Could you check a few things on this model? Use its own coordinates, in mm. A direction names the side the tool comes from. Coordinates: 2 decimals unless noted, no trailing zeros. Write each loop counter-clockwise with the first axis right and the second up, starting at its lowest first coordinate (ties: lowest second). Pieces come first, ordered by that corner, then holes. Notation, with made-up numbers: M 63,70 L 72,70 A26 ccw 72,86 Z; hole C -3,-19 d7. An arc over 180 degrees is marked long. Write item = value, one per line.
```python
from build123d import *

# Parameters (mm, degrees)
F0_W      = 25
F0_H      = 24
F1_DEPTH  = 1
F2_W      = 8
F2_H      = 8
F3_DEPTH  = 4
F5_DEPTH  = 1
F6_R      = 3.0075631212
F6_R_2    = 1.5783263093
F7_DEPTH  = 1
F8_W      = 21
F8_H      = 6
F9_DEPTH  = 3
F10_W     = 17
F10_H     = 0.5
F11_DEPTH = 3
F2_R      = 0.75
F12_DEPTH = 1


with BuildPart() as f1:
    # F0 (on Top) → F1 (new body)
    with BuildSketch(Plane.XY):
        Rectangle(F0_W, F0_H)
    extrude(amount=F1_DEPTH)

    # F2 (on face) → F3 (join)
    with BuildSketch(Plane.XY.offset(1)):
        with Locations((0, 2.5)):
            Rectangle(F2_W, F2_H)
    extrude(amount=F3_DEPTH)

    # F4 (on face) → F5 (cut)
    with BuildSketch(Plane.XY.offset(5)):
        with BuildLine():
            ThreePointArc((0, 6.5), (2.8284271247, 5.3284271247), (4, 2.5))
            Line((4, 2.5), (4, 6.5))
            Line((4, 6.5), (0, 6.5))
        make_face()
        with BuildLine():
            ThreePointArc((-4, 2.5), (-2.8284271247, 5.3284271247), (0, 6.5))
            Line((0, 6.5), (-4, 6.5))
            Line((-4, 6.5), (-4, 2.5))
        make_face()
        with BuildLine():
            Line((-4, -1.5), (0, -1.5))
            ThreePointArc((0, -1.5), (-2.8284271247, -0.3284271247), (-4, 2.5))
            Line((-4, 2.5), (-4, -1.5))
        make_face()
        with BuildLine():
            Line((4, -1.5), (4, 2.5))
            ThreePointArc((4, 2.5), (2.8284271247, -0.3284271247), (0, -1.5))
            Line((0, -1.5), (4, -1.5))
        make_face()
    extrude(amount=-F5_DEPTH, mode=Mode.SUBTRACT)

    # F6 (on face) → F7 (join)
    with BuildSketch(Plane.XY.offset(5)):
        with Locations((0, 2.5)):
            Circle(F6_R)
        with Locations((0, 2.5)):
            Circle(F6_R_2, mode=Mode.SUBTRACT)
    extrude(amount=F7_DEPTH)

    # F8 (on face) → F9 (join)
    with BuildSketch(Plane(origin=(0, 0, 0), x_dir=(1, 0, 0), z_dir=(0, 0, -1))):
        with Locations((0, -9)):
            Rectangle(F8_W, F8_H)
    extrude(amount=F9_DEPTH)

    # F10 (on face) → F11 (join)
    with BuildSketch(Plane(origin=(0, 12, 0), x_dir=(-1, 0, 0), z_dir=(0, 1, 0))):
        with Locations((0, -1.25)):
            Rectangle(F10_W, F10_H)
    extrude(amount=F11_DEPTH)

    # F2 (on face) → F12 (join)
    with BuildSketch(Plane.XY.offset(1)):
        with Locations((-7.5, -7)):
            Circle(F2_R)
    extrude(amount=F12_DEPTH)


solid = f1.part
```
Item 1: If I drill on line 1 along Y through (x, z) = (0, 5.4); line 2 along Y through (x, z) = (0.25, 0.75); line 3 along Z through (x, y) = (-2.25, 1), over which ranges is the centre line in solid material (lowest first)?
Numbers:
line_1 = -0.51 to 0.92, 4.08 to 5.51
line_2 = -12 to 12
line_3 = 0 to 6
Item 2: Imagine slicing it at B-B (y = -7). Write out the boundary of the cut face in (x, z).
Numbers:
outline = M -12.5,0 L 12.5,0 L 12.5,1 L -6.75,1 L -6.75,2 L -8.25,2 L -8.25,1 L -12.5,1 Z
Item 3: Imagine slicing it at D-D (x = 7). Write out the boundary of the cut face in (y, z).
Numbers:
outline = M -12,0 L 6,0 L 6,-3 L 12,-3 L 12,-1.5 L 15,-1.5 L 15,-1 L 12,-1 L 12,1 L -12,1 Z
Item 4: I'm going to push flat-ended pins straight in: P1, Ø10, axis at x = -7.5, y = -9, coming from the +Z side; P2, Ø0.9, axis at y = 2.5, z = 2, coming from the +X side; P3, Ø0.9, axis at x = 3, y = 14, coming from the +Z side. Where does each tip first touch, or does it pass through?
Numbers:
P1 = 2
P2 = 4
P3 = -1
Item 5: For faces 1 (the face through (0, -1.5, 2)), 2 (the face through (10.5, 9, -1)), 3 (the face through (-3, 6, 4)), 4 (the face through (-2, 5, 5)), which set-ups out of +Z, -Z, +X, -X, +Y, -Y let a thin tool reach every point of the face, with its end or its side?
Numbers:
face_1 = +Z, +X, -X, -Y
face_2 = -Z, +X, +Y, -Y
face_3 = +Z, -X, +Y
face_4 = +Z
Item 6: If we mould it in two halves opening along X, with no side actions, what happens to faces 5 (the face through (4, 2, 2)), 6 (the face through (1, 1, 6)), 7 (the face through (0, 3, 5))? For each: pulls with the +X half, pulls with the -X half, needs draft (parallel to the pull), parting line crosses it, or undercut.
Numbers:
face_5 = pulls with the +X half
face_6 = needs draft
face_7 = undercut
Item 7: Imagine slicing it at A-A (x = -7.5). Write out the boundary of the cut face in (y, z), and give its area (3 significant figures).
Numbers:
outline = M -12,0 L 6,0 L 6,-3 L 12,-3 L 12,-1.5 L 15,-1.5 L 15,-1 L 12,-1 L 12,1 L -6.25,1 L -6.25,2 L -7.75,2 L -7.75,1 L -12,1 Z
area = 45.0 mm²
Item 8: Imagine slicing it at C-C (z = -0.5). Write out the boundary of the cut face in (x, y), and give its area (3 significant figures).
Numbers:
outline = M -10.5,6 L 10.5,6 L 10.5,12 L -10.5,12 Z
area = 126 mm²
